Verification items for the finished model (mm, model axes). A direction names the side the tool comes from. Give positions to 0.01 mm unless a question says otherwise; leave off trailing zeros. Write each loop counter-clockwise with the first axis right and the second up, starting at its lowest first coordinate (ties: lowest second). Pieces come first, ordered by that corner, then holes. Notation, with made-up numbers: (58, 54) - (86, 54) arc R5 cw to (86, 60) - close; hole circle Ø10 at (4.25, 23). An arc over 180 degrees is marked (long way). Answer as a JSON object with one key per item and string values. Group by question number.
Item 1: Sectioned sample at B-B, the plane x = -50. Record the boundary of the cut face in (y, z).
Item 2: Go/stop test with flat-tipped pins: pin 1 (9 mm diameter, centred on x = -50, y = -15, fed in from -Z); pin 2 (12 mm diameter, centred on y = -12, z = 22.5, fed in from -X); pin 3 (5 mm diameter, centred on x = -24, y = -26.5, fed in from -Z); pin 4 (15 mm diameter, centred on x = -56, y = -12.5, fed in from +Z). Record where each tip stops, or that it passes through.
Item 3: Sectioned sample at C-C, the plane z = 23. Record the boundary of the cut face in (x, y), and give its area (3 significant figures).
Item 4: Sectioned sample at D-D, the plane y = -7.25. Record the boundary of the cut face in (x, z).
Item 5: Sectioned sample at A-A, the plane y = -15. Record the boundary of the cut face in (x, z).
Item 6: Tool access check on faces 4 (the face through (-35, -15, 18)), 5 (the face through (-28, -8, 35)). Record the directions out of +Z, -Z, +X, -X, +Y, -Y that give a thin tool (end or side, any length) a straight path to the whole face; none if there is none.
Item 7: Scan lines: line 1 along X through (y, z) = (-15.5, 28.5); line 2 along Y through (x, z) = (-17, 4.5); line 3 along X through (y, z) = (-8.5, 8.5). Record each from-to range of solid material in increasing order. Write a range as [from, to].
Item 8: Draft check along Y on faces 1 (the face through (-19, -30, 18)), 2 (the face through (-1, -15, 33)), 3 (the face through (-6.054, -11.396, 17.745)). Enter one of: +Y half, -Y half, draft (parallel to the pull), parting line (faces both ways), or undercut.
```python
from build123d import *

# Parameters (mm, degrees)
F1_DEPTH       = 30
F3_R           = 12
F4_DEPTH       = 35
F5_R           = 5
F7_D           = 5.5
F7_DEPTH       = 16
F7_CSINK_D     = 10
F7_CSINK_ANGLE = 90


with BuildPart() as f1:
    # F0 (on Front) → F1 (new body)
    with BuildSketch(Plane.XZ):
        Polygon((-65, 0), (0, 0), (0, 35), (-35, 35), (-35, 5), (-65, 5), align=None)
    extrude(amount=F1_DEPTH)

    # F3 (on face) → F4 (cut, through all)
    with BuildSketch(Plane.XY.offset(35)):
        with Locations((-17.5, -15)):
            Circle(F3_R)
    extrude(amount=-F4_DEPTH, mode=Mode.SUBTRACT)

    # F5
    f5_edges = [f1.edges().sort_by_distance(p)[0] for p in [
        (0, -15, 35),
        (-35, -15, 35),
    ]]
    fillet(f5_edges, radius=F5_R)

    # F7
    with Locations(Plane(origin=(0, 0, 0), x_dir=(1, 0, 0), z_dir=(0, 0, -1))):
        with Locations((-50, 15)):
            CounterSinkHole(F7_D / 2, F7_CSINK_D / 2, depth=F7_DEPTH, counter_sink_angle=F7_CSINK_ANGLE)


solid = f1.part
```
Geometry check:
{
 "1": {"outline": "(-30, 0) - (-20, 0) - (-17.75, 2.25) - (-17.75, 5) - (-30, 5) - close; (-12.25, 2.25) - (-10, 0) - (0, 0) - (0, 5) - (-12.25, 5) - close"},
 "2": {"pin 1": "z = 0.5", "pin 2": "x = -35", "pin 3": "z = 0", "pin 4": "z = 5"},
 "3": {"outline": "(-35, -30) - (0, -30) - (0, 0) - (-35, 0) - close; hole circle Ø24 at (-17.5, -15)", "area": "598 mm^2"},
 "4": {"outline": "(-65, 0) - (-26.66, 0) - (-26.66, 35) - (-30, 35) arc R5 ccw to (-35, 30) - (-35, 5) - (-65, 5) - close; (-8.34, 0) - (0, 0) - (0, 30) arc R5 ccw to (-5, 35) - (-8.34, 35) - close"},
 "5": {"outline": "(-65, 0) - (-55, 0) - (-52.75, 2.25) - (-52.75, 5) - (-65, 5) - close; (-47.25, 2.25) - (-45, 0) - (-29.5, 0) - (-29.5, 35) - (-30, 35) arc R5 ccw to (-35, 30) - (-35, 5) - (-47.25, 5) - close; (-5.5, 0) - (0, 0) - (0, 30) arc R5 ccw to (-5, 35) - (-5.5, 35) - close"},
 "6": {"face 4": "+Z, -X, +Y, -Y", "face 5": "+Z, +X, -X, +Y, -Y"},
 "7": {"line 1": "[-35, -29.49], [-5.51, 0]", "line 2": "[-30, -26.99], [-3.01, 0]", "line 3": "[-35, -27.59], [-7.41, 0]"},
 "8": {"face 1": "-Y half", "face 2": "draft", "face 3": "undercut"}
}
